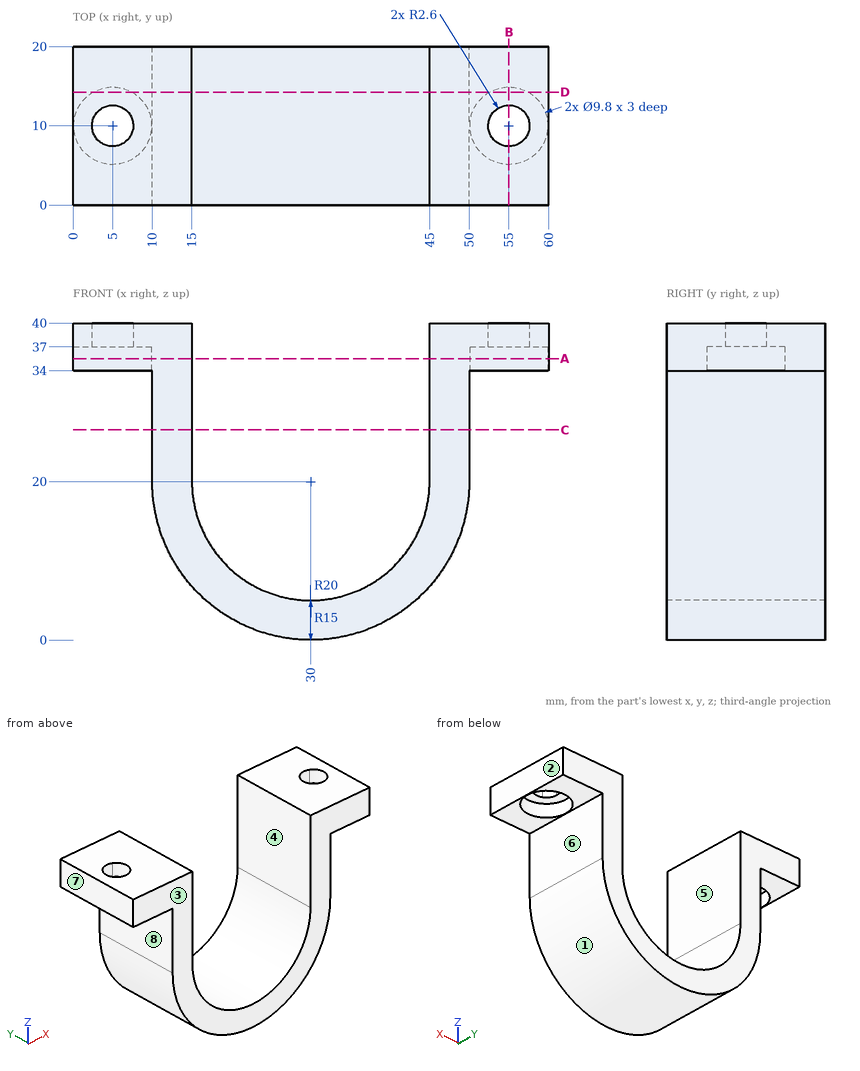
The drawing under review shows one solid part. Ordinate dimensions are in mm from its lowest x, y, z. A direction names the side the tool comes from. Round coordinates to 2 decimals unless told otherwise and drop trailing zeros. Write each loop counter-clockwise with the first axis right and the second up, starting at its lowest first coordinate (ties: lowest second). Pieces come first, ordered by that corner, then holes. Notation, with made-up numbers: (62, 22) - (107, 22) arc R4 cw to (107, 29) - close; hole circle Ø2 at (56, 65.5). An arc over 180 degrees is marked (long way). Write each question's results on one line, items separated by ' | '.
Item 1: Take a section at A-A on z = 35.5. State the section outline as (x, y) points, then the cut area to 3 significant figures.
Calculated:
outline: (0, 0) - (15, 0) - (15, 20) - (0, 20) - close; (45, 0) - (60, 0) - (60, 20) - (45, 20) - close; hole circle Ø9.8 at (5, 10); hole circle Ø9.8 at (55, 10) | area: 449 mm^2
Item 2: To check wall thickness, follow line 1 along X through (y, z) = (16, 32); line 2 along Y through (x, z) = (55, 35.5); line 3 along X through (y, z) = (2.5, 9). State the ranges of each line that lie inside material, in increasing order. Write a range as from..to.
Calculated:
line 1: x = 10..15, 45..50 | line 2: y = 0..5.1, 14.9..20 | line 3: x = 13.3..19.8, 40.2..46.7
Item 3: Draft analysis for pull direction X (two halves, no side actions). For the marked faces 1, 2, 3 and 4, state which applies: pulls with the +X half, pulls with the -X half, needs draft (parallel to the pull), parting line crosses it, or undercut.
Calculated:
face 1: parting line crosses it | face 2: pulls with the +X half | face 3: needs draft | face 4: undercut
Item 4: Take a section at D-D on y = 14.25. State the section outline as (x, z) points, then the cut area to 3 significant figures.
Calculated:
outline: (0, 34) - (2.56, 34) - (2.56, 37) - (7.44, 37) - (7.44, 34) - (10, 34) - (10, 20) arc R20 ccw to (50, 20) - (50, 34) - (52.56, 34) - (52.56, 37) - (57.44, 37) - (57.44, 34) - (60, 34) - (60, 40) - (45, 40) - (45, 20) arc R15 cw to (15, 20) - (15, 40) - (0, 40) - close | area: 566 mm^2
Item 5: For the marked faces 5, 6, 7 and 8, list the 3-axis set-ups (+Z, -Z, +X, -X, +Y, -Y) from which the entire face can be reached by the end or side of a thin tool; tool diameter is ignored.
Calculated:
face 5: +Z, +Y, -Y | face 6: -Z, +X, +Y, -Y | face 7: +Z, -Z, -X, +Y, -Y | face 8: -Z, -X, +Y, -Y
Item 6: For pin 1 (4 mm diameter, centred on y = 2.5, z = 16, fed in from +X); pin 2 (2 mm diameter, centred on x = 8, y = 16.5, fed in from -Z); pin 3 (6 mm diameter, centred on y = 4, z = 30, fed in from +X), all flat-tipped, find the tip position at first contact; note any pin that passes through.
Calculated:
pin 1: stops at x = 49.9 | pin 2: stops at z = 34 | pin 3: stops at x = 50
Item 7: Take a section at C-C on z = 26.5. State the section outline as (x, y) points, then the cut area to 3 significant figures.
Calculated:
outline: (10, 0) - (15, 0) - (15, 20) - (10, 20) - close; (45, 0) - (50, 0) - (50, 20) - (45, 20) - close | area: 200 mm^2
Item 8: Take a section at B-B on x = 55. State the section outline as (y, z) points, then the cut area to 3 significant figures.
Calculated:
outline: (0, 34) - (5.1, 34) - (5.1, 37) - (7.4, 37) - (7.4, 40) - (0, 40) - close; (12.6, 37) - (14.9, 37) - (14.9, 34) - (20, 34) - (20, 40) - (12.6, 40) - close | area: 75.0 mm^2
